Geometry: final body of the model. Coordinates: model frame, mm. A direction names the side the tool comes from. Give positions to 0.01 mm unless a question says otherwise; leave off trailing zeros. Loops run counter-clockwise (first coordinate to the right, second up) from the corner with the lowest first, then second, coordinate; pieces in that order, holes last. Notation, with made-up numbers: (80, 67) -> (109, 67) arc R20 cw to (109, 92) -> close; hole circle Ø6 at (79, -17.75). An arc over 180 degrees is marked (long way). Answer in a Markdown table with one row per item. Add a question column.
1) Section query D-D (y = 0.3). Return the cut outline in (x, z).
2) Section query B-B (x = 12.25). Return the cut outline in (y, z), plus the area to 3 significant figures.
3) Draft query along X for faces 5 (the flat face through (-15, 1, -10)), 6 (the flat face through (-5.5, 1, -18)), 7 (the flat face through (0, 0, -10)). Return one class per face: +X half, -X half, draft (parallel to the pull), parting line (faces both ways), or undercut.
4) Section query A-A (z = -17). Return the cut outline in (x, y).
5) Access query for faces 1 (the cylindrical face through (-13.49, 0.79, -17.39)), 2 (the flat face through (-12, 1, -20)), 3 (the cylindrical face through (9.801, 0.811, -19.715)), 4 (the flat face through (12, 1, -20)). Directions: +Z, -Z, +X, -X, +Y, -Y. A direction counts if a zero-diameter tool reaches every point of the face in a straight line with its end or side. Return the directions, or none.
6) Line query: line 1 (X direction, y = 1.45, z = -17); line 2 (Z direction, x = 12.25, y = 0.95); line 3 (X direction, y = 0.8, z = -17.5). Output: solid intervals per line, ascending. Write a range as from..to.
7) First-contact query: P1, Ø1.6, axis at x = 12.25, z = -17, coming from the -Y side; P2, Ø0.5, axis at x = 7, y = 1, coming from the -Z side. Flat tips, straight axial feed; report the tip coordinate or a pass-through.
8) Section query C-C (z = -3). Return the cut outline in (x, y), plus the area to 3 significant figures.
```python
from build123d import *

# Parameters (mm, degrees)
BOSS_EXTRUDE1_DEPTH      = 1.6
FILLET1_R                = 1
M2_CLEARANCE_HOLE1_D     = 2.6
M2_CLEARANCE_HOLE1_DEPTH = 1.6
M2_CLEARANCE_HOLE1_TIP   = 0.781118805
FILLET2_R                = 0.5


with BuildPart() as part:
    # Sketch1 → Boss-Extrude1 (new body)
    with BuildSketch(Plane(origin=(0, 0, 0), x_dir=(1, 0, 0), z_dir=(0, 1, 0))):
        Polygon((-15, 20), (-15, 0), (15, 0), (15, 20), (9.5, 20), (9.5, 11.5), (5.5, 11.5), (5.5, 25), (-5.5, 25), (-5.5, 11.5), (-9.5, 11.5), (-9.5, 20), align=None)
    extrude(amount=BOSS_EXTRUDE1_DEPTH)

    # Fillet1
    fillet1_edges = [part.edges().sort_by_distance(p)[0] for p in [
        (-9.5, 0.8, -20),
        (-9.5, 0.8, -11.5),
        (-5.5, 0.8, -25),
        (5.5, 0.8, -25),
        (9.5, 0.8, -11.5),
        (9.5, 0.8, -20),
        (15, 0.8, -20),
        (15, 0.8, 0),
        (-15, 0.8, 0),
        (-15, 0.8, -20),
    ]]
    fillet(fillet1_edges, radius=FILLET1_R)

    # M2 Clearance Hole1
    with Locations(Plane(origin=(0, 1.6, 0), x_dir=(1, 0, 0), z_dir=(0, 1, 0))):
        with Locations((-12.25, 17), (-12.25, 3), (12.25, 3), (12.25, 17)):
            Hole(M2_CLEARANCE_HOLE1_D / 2, depth=M2_CLEARANCE_HOLE1_DEPTH)
            with Locations((0, 0, -(M2_CLEARANCE_HOLE1_DEPTH + M2_CLEARANCE_HOLE1_TIP / 2))):  # 118° drill point
                Cone(0, M2_CLEARANCE_HOLE1_D / 2, M2_CLEARANCE_HOLE1_TIP, mode=Mode.SUBTRACT)

    # Fillet2
    fillet2_edges = [part.edges().sort_by_distance(p)[0] for p in [
        (-5.5, 0.8, -11.5),
        (5.5, 0.8, -11.5),
    ]]
    fillet(fillet2_edges, radius=FILLET2_R)


solid = part.part
```
Evaluation:
| question | item | result |
|---|---|---|
| 1 | outline | (-15, -19) arc R1 ccw to (-14, -20) -> (-10.5, -20) arc R1 ccw to (-9.5, -19) -> (-9.5, -12.5) arc R1 cw to (-8.5, -11.5) -> (-6, -11.5) arc R0.5 cw to (-5.5, -12) -> (-5.5, -24) arc R1 ccw to (-4.5, -25) -> (4.5, -25) arc R1 ccw to (5.5, -24) -> (5.5, -12) arc R0.5 cw to (6, -11.5) -> (8.5, -11.5) arc R1 cw to (9.5, -12.5) -> (9.5, -19) arc R1 ccw to (10.5, -20) -> (14, -20) arc R1 ccw to (15, -19) -> (15, -1) arc R1 ccw to (14, 0) -> (-14, 0) arc R1 ccw to (-15, -1) -> close; hole circle Ø2.6 at (-12.25, -17); hole circle Ø2.6 at (-12.25, -3); hole circle Ø2.6 at (12.25, -17); hole circle Ø2.6 at (12.25, -3) |
| 2 | outline | (0, -20) -> (1.6, -20) -> (1.6, -18.3) -> (0, -18.3) -> close; (0, -15.7) -> (1.6, -15.7) -> (1.6, -4.3) -> (0, -4.3) -> close; (0, -1.7) -> (1.6, -1.7) -> (1.6, 0) -> (0, 0) -> close |
| 2 | area | 23.7 mm² |
| 3 | face 5 | -X half |
| 3 | face 6 | undercut |
| 3 | face 7 | draft |
| 4 | outline | (-15, 0) -> (-13.55, 0) -> (-13.55, 1.6) -> (-15, 1.6) -> close; (-10.95, 0) -> (-9.5, 0) -> (-9.5, 1.6) -> (-10.95, 1.6) -> close; (-5.5, 0) -> (5.5, 0) -> (5.5, 1.6) -> (-5.5, 1.6) -> close; (9.5, 0) -> (10.95, 0) -> (10.95, 1.6) -> (9.5, 1.6) -> close; (13.55, 0) -> (15, 0) -> (15, 1.6) -> (13.55, 1.6) -> close |
| 5 | face 1 | +Y, -Y |
| 5 | face 2 | -Z, -X, +Y, -Y |
| 5 | face 3 | -Z, +Y, -Y |
| 5 | face 4 | -Z, +X, +Y, -Y |
| 6 | line 1 | -15..-13.55, -10.95..-9.5, -5.5..5.5, 9.5..10.95, 13.55..15 |
| 6 | line 2 | -20..-18.3, -15.7..-4.3, -1.7..0 |
| 6 | line 3 | -15..-13.45, -11.05..-9.5, -5.5..5.5, 9.5..11.05, 13.45..15 |
| 7 | P1 | through |
| 7 | P2 | z = -11.5 |
| 8 | outline | (-15, 0) -> (-13.55, 0) -> (-13.55, 1.6) -> (-15, 1.6) -> close; (-10.95, 0) -> (10.95, 0) -> (10.95, 1.6) -> (-10.95, 1.6) -> close; (13.55, 0) -> (15, 0) -> (15, 1.6) -> (13.55, 1.6) -> close |
| 8 | area | 39.7 mm² |
